from build123d import *

# Parameters (mm, degrees)
BOSS_EXTRUDE1_DEPTH = 50
CUT_EXTRUDE1_DEPTH  = 50
SKETCH3_R           = 7.5
BOSS_EXTRUDE2_DEPTH = 150
FILLET1_R           = 10


with BuildPart() as part:
    # Sketch1 → Boss-Extrude1 (new body)
    with BuildSketch(Plane(origin=(0, 0, 0), x_dir=(1, 0, 0), z_dir=(0, 1, 0))):
        Polygon((0, 0), (0, 70), (20, 70), (20, 20), (70, 20), (70, 0), align=None)
    extrude(amount=BOSS_EXTRUDE1_DEPTH)

    # Sketch2 → Cut-Extrude1 (cut)
    with BuildSketch(Plane(origin=(0, 50, 0), x_dir=(1, 0, 0), z_dir=(0, 1, 0))):
        Polygon((0, 17.6), (17.754999296, 0), (0, 0), align=None)
    extrude(amount=-CUT_EXTRUDE1_DEPTH, mode=Mode.SUBTRACT)

    # Sketch3 → Boss-Extrude2 (add)
    with BuildSketch(Plane(origin=(8.799661731, 0, -8.8771584), x_dir=(0.7101999718389179, 0, 0.7040000000000001), z_dir=(-0.7040000000000001, 0, 0.7101999718389179))):
        with Locations((0.1096, 35)):
            Circle(SKETCH3_R)
        with Locations(Location((0.1096, 15, 0), (0, 0, 180))):
            Circle(SKETCH3_R)
    extrude(amount=BOSS_EXTRUDE2_DEPTH)

    # Fillet1
    fillet1_edges = [part.edges().sort_by_distance(p)[0] for p in [
        (20, 25, -70),
        (70, 25, -20),
    ]]
    fillet(fillet1_edges, radius=FILLET1_R)


solid = part.part
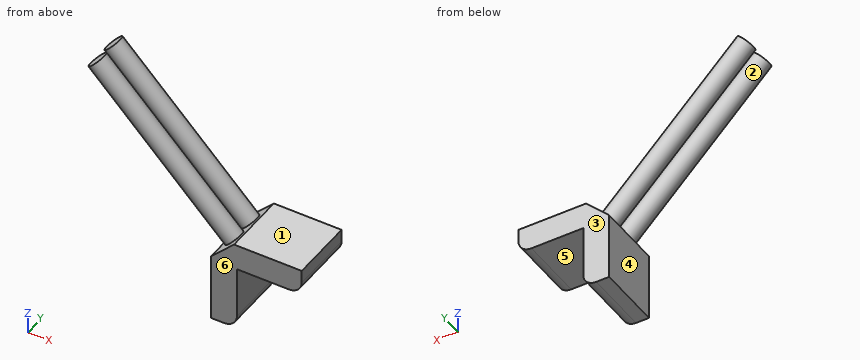
Work out the finished part from the listing and answer in its coordinate system (mm). Face numbers are marked on the shaded views. A direction names the side the tool comes from. Round coordinates to 2 decimals unless told otherwise and drop trailing zeros. Order: outer loops, then holes, each group sorted by start corner. A loop starts at its lowest first (then second) coordinate and runs counter-clockwise, first axis right, second up. Notation, with made-up numbers: M 58.25,59.5 L 99.25,59.5 A16 ccw 99.25,70.5 Z; hole C -12.5,-34 d1. An arc over 180 degrees is marked long. One line per item, written item: value.
Q1. Find section C-C on x = 29. Write down the section's boundary in (y, z), then the cut area to 3 significant figures.
Derived:
outline: M 0,-20 L 50,-20 L 50,0 L 0,0 Z
area: 1,000 mm²
Q2. Find section D-D on y = 38.5. Write down the section's boundary in (x, z) (3 decimals).
Derived:
outline: M -101.433,93.06 L 4.167,-13.47 L 0,-17.6 L 0,-70 L 10,-70 A10 ccw 20,-60 L 20,-20 L 60,-20 A10 ccw 70,-10 L 70,0 L 17.755,0 L 13.588,-4.13 L -92.012,102.4 Z
Q3. Straight lines are drawn through the part: line 1 (X direction, y = 14.5, z = -22.5); line 2 (Y direction, x = -63.5, z = 65); line 3 (Z direction, x = 53.5, y = 24). For each, find the intervals that lie inside material, in ascending order.
Derived:
line 1: 0 to 20
line 2: 7.52 to 22.48, 27.52 to 42.48
line 3: -20 to 0
Q4. Find section B-B on z = -25. Write down the section's boundary in (x, y).
Derived:
outline: M 0,0 L 20,0 L 20,50 L 0,50 Z
Q5. Flat-ended cylindrical pins translate along their axes: pin 1 (4 mm diameter, centred on y = 27, z = 3, fed in from +X); pin 2 (2 mm diameter, centred on y = 37.5, z = 13, fed in from +X); pin 3 (15 mm diameter, centred on x = 42.5, y = 13.5, fed in from +Z). Find the tip coordinate at first contact, or state that the pin passes through.
Derived:
pin 1: x = 3.99
pin 2: x = -1.69
pin 3: z = 0
Q6. Determine the mould class of the marked faces 1, 2 and 3 for opening direction Y: released by +Y, released by -Y, zero draft, split by the parting line, or undercut.
Derived:
face 1: zero draft
face 2: undercut
face 3: released by +Y
Q7. Find section A-A on y = 4.5. Write down the section's boundary in (x, z) (3 decimals), then the cut area to 3 significant figures.
Derived:
outline: M 0,-70 L 10,-70 A10 ccw 20,-60 L 20,-20 L 60,-20 A10 ccw 70,-10 L 70,0 L 17.755,0 L 0,-17.6 Z
area: 2,200 mm²
Q8. For the marked faces 4, 5 and 6, determine the directions among +Z, -Z, +X, -X, +Y, -Y from which every point of the face is accessible in a straight line to the end or side of a thin tool.
Derived:
face 4: -Z, -X, +Y, -Y
face 5: -Z, +X, +Y, -Y
face 6: +Z, -Z, +X, -X, -Y
